Source: three-view drawing plus pictorial views. Frame: mm from the lowest corner of the part. A direction names the side the tool comes from. Give positions to 0.01 mm unless a question says otherwise; leave off trailing zeros. Order: outer loops, then holes, each group sorted by start corner. A loop starts at its lowest first (then second) coordinate and runs counter-clockwise, first axis right, second up.
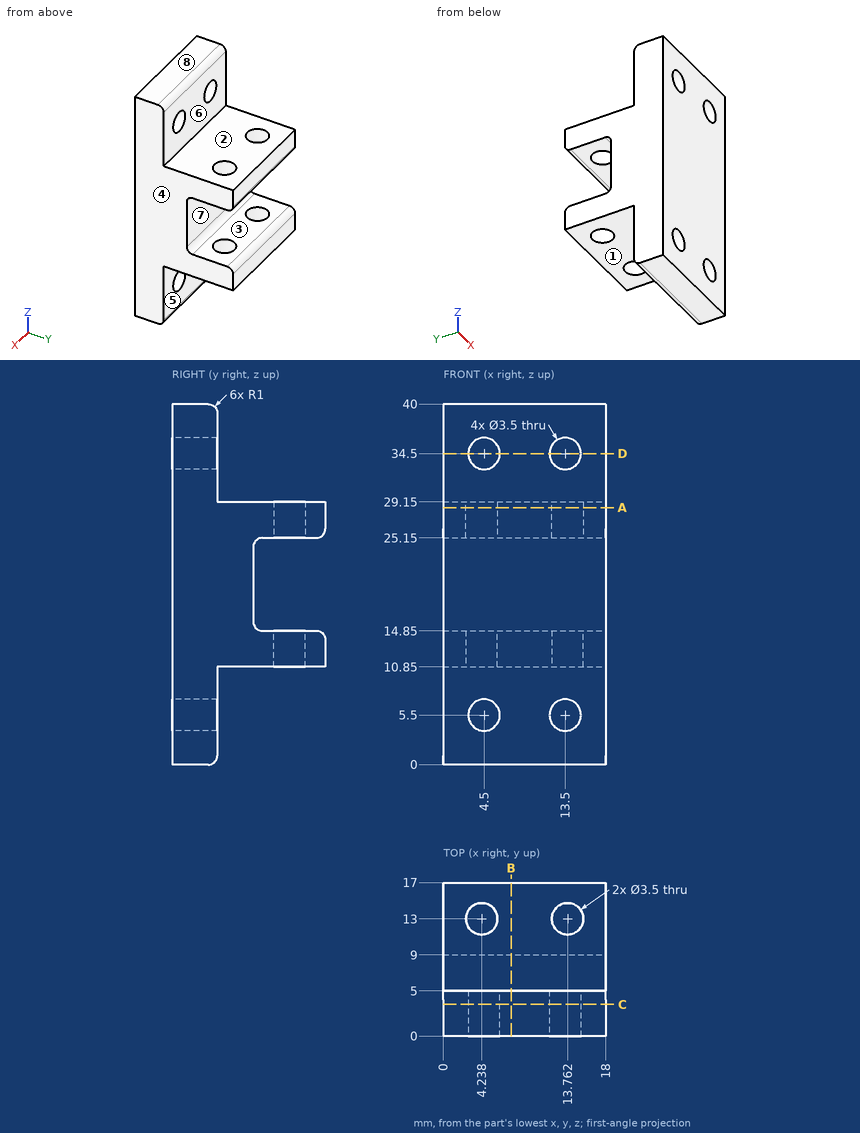
1) Section query D-D on z = 34.5. Output: boundary loops of the cut face in (x, y).
Checks:
outline: (0, 0) - (2.75, 0) - (2.75, 5) - (0, 5) - close; (6.25, 0) - (11.75, 0) - (11.75, 5) - (6.25, 5) - close; (15.25, 0) - (18, 0) - (18, 5) - (15.25, 5) - close
2) Section query C-C on y = 3.5. Output: boundary loops of the cut face in (x, z), and give its area (3 significant figures).
Checks:
outline: (0, 0) - (18, 0) - (18, 40) - (0, 40) - close; hole circle Ø3.5 at (4.5, 5.5); hole circle Ø3.5 at (4.5, 34.5); hole circle Ø3.5 at (13.5, 5.5); hole circle Ø3.5 at (13.5, 34.5)
area: 682 mm2
3) Reachability of the marked faces 5, 6, 7 and 8 from +Z, -Z, +X, -X, +Y, -Y: full face, straight path, thin tool, end or side. Return the list, or none.
Checks:
face 5: -Z, +X, -X, +Y
face 6: +Z, +X, -X, +Y
face 7: +X, -X, +Y
face 8: +Z, +X, -X, +Y, -Y
4) First-contact query: pin 1 Ø6.5 at (x, y) = (5.5, 13.5) entering from +Z; pin 2 Ø5.5 at (x, z) = (4.5, 5.5) entering from +Y; pin 3 Ø3.5 at (x, y) = (7, 10.5) entering from -Z. Flat tips, straight axial feed; report the tip coordinate or a pass-through.
Checks:
pin 1: stops at z = 29.15
pin 2: stops at y = 5
pin 3: stops at z = 10.85
5) Ray query, L1, parallel to Z at x = 4.5, y = 1.5; L2, parallel to Z at x = 6, y = 15.5; L3, parallel to X at y = 13, z = 13.55. Return the intervals inside material, ascending.
Checks:
L1: z = 0 to 3.75, 7.25 to 32.75, 36.25 to 40
L2: z = 10.85 to 14.85, 25.15 to 29.15
L3: x = 0 to 2.49, 5.99 to 12.01, 15.51 to 18
6) Pull-direction query (Z, two-part tool) for the marked faces 1, 2, 3 and 4; classes: +Z half, -Z half, draft (parallel to the pull), parting line (faces both ways), or undercut.
Checks:
face 1: -Z half
face 2: +Z half
face 3: undercut
face 4: draft
7) Section query A-A on z = 28.5. Output: boundary loops of the cut face in (x, y), and give its area (3 significant figures).
Checks:
outline: (0, 0) - (18, 0) - (18, 17) - (0, 17) - close; hole circle Ø3.5 at (4.24, 13); hole circle Ø3.5 at (13.76, 13)
area: 287 mm2
8) Section query B-B on x = 7.5. Output: boundary loops of the cut face in (y, z), and give its area (3 significant figures).
Checks:
outline: (0, 0) - (4, 0) arc R1 ccw to (5, 1) - (5, 10.85) - (17, 10.85) - (17, 13.85) arc R1 ccw to (16, 14.85) - (10, 14.85) arc R1 cw to (9, 15.85) - (9, 24.15) arc R1 cw to (10, 25.15) - (16, 25.15) arc R1 ccw to (17, 26.15) - (17, 29.15) - (5, 29.15) - (5, 39) arc R1 ccw to (4, 40) - (0, 40) - close
area: 337 mm2
